Geometry: final body of the model. Coordinates: model frame, mm. Face numbers are marked on the shaded views. A direction names the side the tool comes from. Round coordinates to 2 decimals unless told otherwise and drop trailing zeros. Loops run counter-clockwise (first coordinate to the right, second up) from the corner with the lowest first, then second, coordinate; pieces in that order, holes last. Notation, with made-up numbers: M -29,-28 L 4,-28 A28 ccw 4,-2 Z; hole C 25,-9 d3. An arc over 180 degrees is marked long. Answer as a JSON object with one key per item and string values.
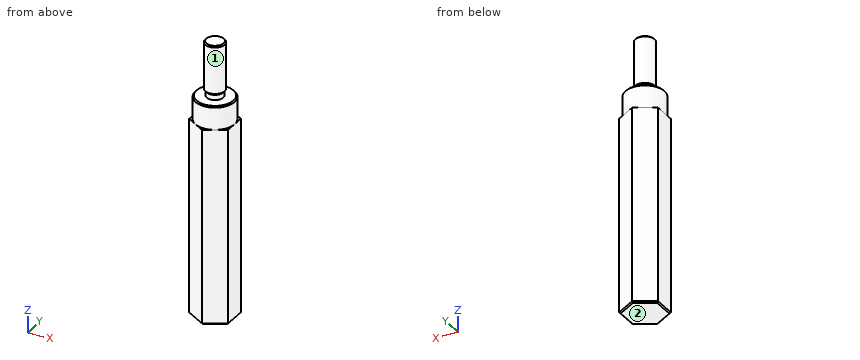
```python
from build123d import *

# Parameters (mm, degrees)
AUFSATZ_LINEAR_AUSTRAGEN1_DEPTH = 70
FASE1_SIZE                      = 0.3
FASE2_SIZE                      = 0.3


with BuildPart() as part:
    # Skizze1 → Aufsatz-Linear austragen1 (new body)
    with BuildSketch(Plane.XY):
        Polygon((0, 5.773502692), (-5, 2.886751346), (-5, -2.886751346), (0, -5.773502692), (5, -2.886751346), (5, 2.886751346), align=None)
    extrude(amount=AUFSATZ_LINEAR_AUSTRAGEN1_DEPTH)

    # Skizze2 → Schnitt-Rotation1 (revolve, cut)
    with BuildSketch(Plane(origin=(0, 0, 0), x_dir=(0, 0, -1), z_dir=(1, 0, 0)), mode=Mode.PRIVATE) as schnitt_rotation1_sk:
        Polygon((-70, 2.5), (-56, 2.5), (-56, 5), (-50, 5), (-50, 7.5), (-70, 7.5), align=None)
    revolve(schnitt_rotation1_sk.sketch.rotate(Axis((0, 0, 56.716665977), (0, 0, 1)), 90), axis=Axis((0, 0, 56.716665977), (0, 0, 1)), mode=Mode.SUBTRACT)

    # Fase1
    fase1_edges = [part.edges().sort_by_distance(p)[0] for p in [
        (2.5, 0, 70),
        (5, 0, 56),
    ]]
    chamfer(fase1_edges, length=FASE1_SIZE)

    # Skizze3 → Schnitt-Rotation2 (revolve, cut)
    with BuildSketch(Plane(origin=(0, 0, 0), x_dir=(0, 0, -1), z_dir=(1, 0, 0)), mode=Mode.PRIVATE) as schnitt_rotation2_sk:
        Polygon((-56, 2.5), (-57.8, 2.5), (-57.323298563, 2.1), (-56, 2.1), align=None)
    revolve(schnitt_rotation2_sk.sketch.rotate(Axis((0, 0, 56), (0, 0, 1)), 90), axis=Axis((0, 0, 56), (0, 0, 1)), mode=Mode.SUBTRACT)

    # Fase2
    fase2_edges = [part.edges().sort_by_distance(p)[0] for p in [
        (5, 0, 0),
        (2.5, -4.330127019, 0),
        (-2.5, -4.330127019, 0),
        (-5, 0, 0),
        (-2.5, 4.330127019, 0),
        (2.5, 4.330127019, 0),
    ]]
    chamfer(fase2_edges, length=FASE2_SIZE)


solid = part.part
```
1) Line query: probe 1 along Y at (x, z) = (0.25, 58.5); probe 2 along Z at (x, y) = (4.5, 2.5). Output: solid intervals per line, ascending.
Geometry results:
{"probe 1": "-2.49 to 2.49", "probe 2": "0 to 50"}
2) Set-up query: the marked faces 1 and 2. Return all of +Z, -Z, +X, -X, +Y, -Y with unobstructed straight access to the full face (end or side cutting, diameter ignored); none if empty.
Geometry results:
{"face 1": "+Z", "face 2": "-Z, +X, -X, +Y, -Y"}
3) First-contact query: pin 1 (1 mm diameter, centred on x = -2, z = 57.5, fed in from -Y); pin 2 (2.5 mm diameter, centred on x = 3.5, y = 3, fed in from +Z); pin 3 (1 mm diameter, centred on y = -2.5, z = 54, fed in from -X). Flat tips, straight axial feed; report the tip coordinate or a pass-through.
Geometry results:
{"pin 1": "y = -1.92", "pin 2": "z = 56", "pin 3": "x = -4.58"}
4) Cut plane A-A on z = 34. Return the cut outline in (x, y).
Geometry results:
{"outline": "M -5,-2.89 L 0,-5.77 L 5,-2.89 L 5,2.89 L 0,5.77 L -5,2.89 Z"}
